from build123d import *

# Parameters (mm, degrees)
F0_R     = 2.54
F1_DEPTH = 2.65684


with BuildPart() as f1:
    # F0 (on Front) → F1 (new body)
    with BuildSketch(Plane.XZ):
        with BuildLine():
            Line((-69.85, 0), (0, 0))
            Line((0, 0), (69.85, 0))
            ThreePointArc((69.85, 0), (74.340128, 1.859872), (76.2, 6.35))
            Line((76.2, 6.35), (76.2, 69.85))
            ThreePointArc((76.2, 69.85), (74.340128, 74.340128), (69.85, 76.2))
            Line((69.85, 76.2), (24.796671, 76.2))
            ThreePointArc((24.796671, 76.2), (20.535787, 77.841776), (18.478185, 81.918151))
            Line((18.478185, 81.918151), (13.271815, 133.981849))
            ThreePointArc((13.271815, 133.981849), (11.214213, 138.058224), (6.953329, 139.7))
            Line((6.953329, 139.7), (0, 139.7))
            Line((0, 139.7), (-6.953329, 139.7))
            ThreePointArc((-6.953329, 139.7), (-11.214213, 138.058224), (-13.271815, 133.981849))
            Line((-13.271815, 133.981849), (-18.478185, 81.918151))
            ThreePointArc((-18.478185, 81.918151), (-20.535787, 77.841776), (-24.796671, 76.2))
            Line((-24.796671, 76.2), (-69.85, 76.2))
            ThreePointArc((-69.85, 76.2), (-74.340128, 74.340128), (-76.2, 69.85))
            Line((-76.2, 69.85), (-76.2, 6.35))
            ThreePointArc((-76.2, 6.35), (-74.340128, 1.859872), (-69.85, 0))
        make_face()
        with Locations((-69.85, 6.35)):
            Circle(F0_R, mode=Mode.SUBTRACT)
        with Locations((-35.147801, 21.569327)):
            Circle(F0_R, mode=Mode.SUBTRACT)
        with Locations((-35.147801, 53.738443)):
            Circle(F0_R, mode=Mode.SUBTRACT)
        with Locations((35.147801, 21.569327)):
            Circle(F0_R, mode=Mode.SUBTRACT)
        with Locations((69.85, 6.35)):
            Circle(F0_R, mode=Mode.SUBTRACT)
        with Locations((35.147801, 53.738443)):
            Circle(F0_R, mode=Mode.SUBTRACT)
        with Locations((-69.85, 69.85)):
            Circle(F0_R, mode=Mode.SUBTRACT)
        with Locations((69.85, 69.85)):
            Circle(F0_R, mode=Mode.SUBTRACT)
        with BuildLine():
            Line((-6.35, 106.68), (-6.35, 127))
            ThreePointArc((-6.35, 127), (0, 133.35), (6.35, 127))
            Line((6.35, 127), (6.35, 106.68))
            ThreePointArc((6.35, 106.68), (0, 100.33), (-6.35, 106.68))
        make_face(mode=Mode.SUBTRACT)
    extrude(amount=F1_DEPTH)


solid = f1.part
Source: CAD feature listing. Evaluate the final solid. Frame: model axes, mm. A direction names the side the tool comes from. Round coordinates to 2 decimals unless told otherwise and drop trailing zeros. Loops run counter-clockwise (first coordinate to the right, second up) from the corner with the lowest first, then second, coordinate; pieces in that order, holes last. Notation, with made-up numbers: (10.5, -34) - (55.5, -34) arc R22 ccw to (55.5, 1) - close; hole circle Ø10 at (-38.5, 87). An arc over 180 degrees is marked (long way). Write item = value, one per line. Start each with the question number.
(1) Ray query, line 1 along Z through (x, y) = (-69.85, -1.9); line 2 along X through (y, z) = (-0.85, 54); line 3 along Z through (x, y) = (-68, -0.9). Return the intervals inside material, ascending. Write a range as from..to.
(2) Section query D-D, the plane x = -28.5. Output: boundary loops of the cut face in (y, z), plus the area to 3 significant figures.
(3) Section query C-C, the plane y = -1.4. State how many separate pieces and enclosed holes the cut face has, plus the area to 3 significant figures.
(4) Set-up query: faces 5 (the face through (-1, 0, 40)), 6 (the face through (-0.14, -1.31, 133.35)). Return all of +Z, -Z, +X, -X, +Y, -Y with unobstructed straight access to the full face (end or side cutting, diameter ignored); none if empty.
(5) Section query B-B, the plane x = 0. Output: boundary loops of the cut face in (y, z), plus the area to 3 significant figures.
(6) Section query A-A, the plane z = 124. Output: boundary loops of the cut face in (x, y).
(7) Pin query (flat end, axial travel): pin 1 (3 mm diameter, centred on x = -35.15, z = 53.74, fed in from -Y); pin 2 (1.3 mm diameter, centred on x = -58, y = -1.5, fed in from +Z); pin 3 (0.8 mm diameter, centred on y = -2, z = 118.5, fed in from +X). Return the tip coordinate at first contact, or that it passes through.
(8) Pull-direction query (Z, two-part tool) for faces 1 (the face through (74.29, -1.31, 1.81)), 2 (the face through (74.39, -1.31, 74.29)), 3 (the face through (37.494, -1.31, 20.596)), 4 (the face through (-72.388, -1.31, 6.462)); classes: +Z half, -Z half, draft (parallel to the pull), parting line (faces both ways), or undercut.
Conclusion:
q1.line_1 = 0..3.81, 8.89..67.31, 72.39..76.2
q1.line_2 = -76.2..-37.67, -32.62..32.62, 37.67..76.2
q1.line_3 = 0..4.61, 8.09..68.11, 71.59..76.2
q2.outline = (-2.66, 0) - (0, 0) - (0, 76.2) - (-2.66, 76.2) - close
q2.area = 202 mm2
q3.separate_pieces = 1
q3.enclosed_holes = 9
q3.area = 13,000 mm2
q4.face_5 = +Z, -Z, +X, -X, +Y
q4.face_6 = +Y, -Y
q5.outline = (-2.66, 0) - (0, 0) - (0, 100.33) - (-2.66, 100.33) - close; (-2.66, 133.35) - (0, 133.35) - (0, 139.7) - (-2.66, 139.7) - close
q5.area = 283 mm2
q6.outline = (-14.27, -2.66) - (-6.35, -2.66) - (-6.35, 0) - (-14.27, 0) - close; (6.35, -2.66) - (14.27, -2.66) - (14.27, 0) - (6.35, 0) - close
q7.pin_1 = through
q7.pin_2 = 76.2
q7.pin_3 = 14.86
q8.face_1 = -Z half
q8.face_2 = +Z half
q8.face_3 = undercut
q8.face_4 = undercut
